Design review of the part shown in the three views and the two pictorial views. Dimensions are in mm from the part's minimum x, y and z. A direction names the side the tool comes from. Round coordinates to 2 decimals unless told otherwise and drop trailing zeros. Order: outer loops, then holes, each group sorted by start corner. A loop starts at its lowest first (then second) coordinate and runs counter-clockwise, first axis right, second up.
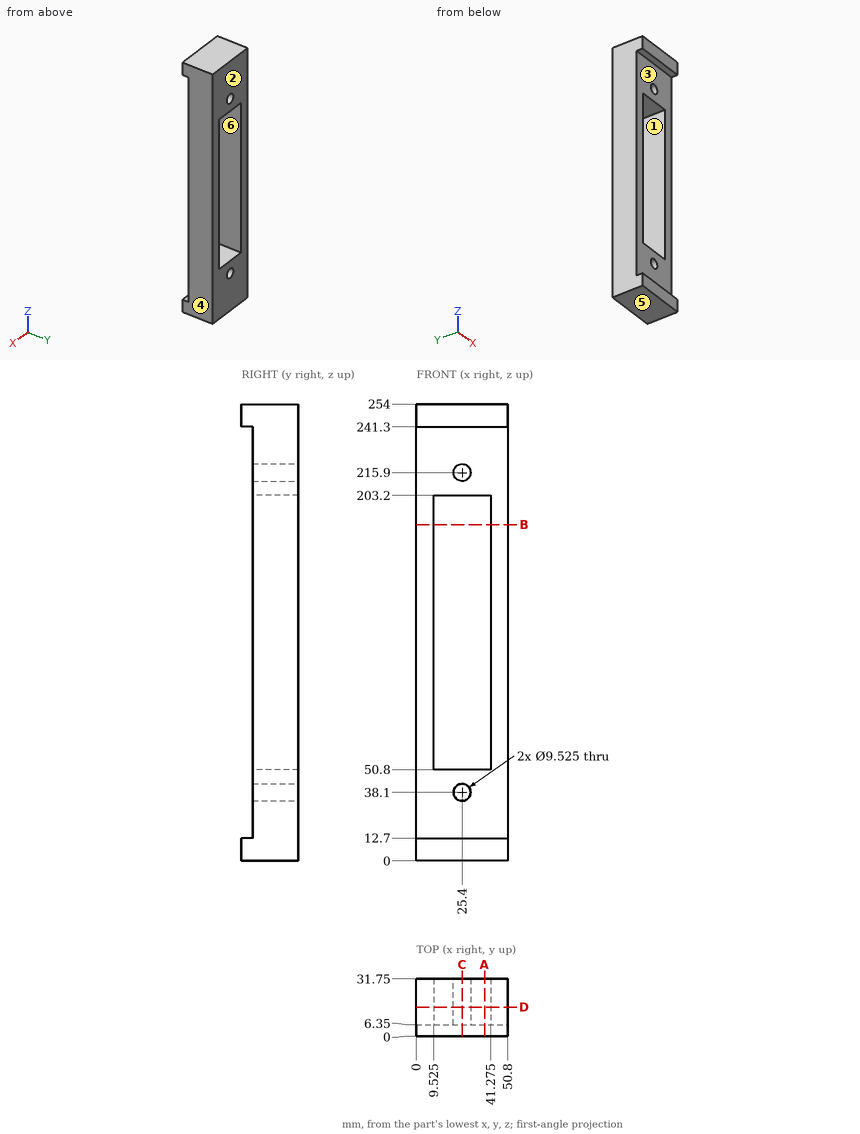
(1) Consider section B-B (z = 187). Write out the cut boundary in (x, y) (3 decimals).
Data:
outline: (0, 6.35) - (9.525, 6.35) - (9.525, 31.75) - (0, 31.75) - close; (41.275, 6.35) - (50.8, 6.35) - (50.8, 31.75) - (41.275, 31.75) - close
(2) To check wall thickness, follow probe 1 along Z at (x, y) = (25, 13); probe 2 along Z at (x, y) = (25.4, 17); probe 3 along Z at (x, y) = (16, 9.5). State the ranges of each line that lie inside material, in increasing order.
Data:
probe 1: z = 0 to 33.35, 42.85 to 50.8, 203.2 to 211.15, 220.65 to 254
probe 2: z = 0 to 33.34, 42.86 to 50.8, 203.2 to 211.14, 220.66 to 254
probe 3: z = 0 to 50.8, 203.2 to 254
(3) Draft analysis for pull direction Z (two halves, no side actions). For the marked faces 4, 5 and 6, state which applies: pulls with the +Z half, pulls with the -Z half, needs draft (parallel to the pull), parting line crosses it, or undercut.
Data:
face 4: needs draft
face 5: pulls with the -Z half
face 6: undercut
(4) Consider section D-D (y = 16). Write out the cut boundary in (x, z) (1 decimal), and give its area (3 significant figures).
Data:
outline: (0, 0) - (50.8, 0) - (50.8, 254) - (0, 254) - close; hole (9.5, 50.8) - (41.3, 50.8) - (41.3, 203.2) - (9.5, 203.2) - close; hole circle Ø9.5 at (25.4, 38.1); hole circle Ø9.5 at (25.4, 215.9)
area: 7,920 mm2
(5) Insertion check: pin 1 (12.5 mm diameter, centred on x = 25.4, z = 215.9, fed in from -Y); pin 2 (8.5 mm diameter, centred on x = 25.4, z = 38.1, fed in from -Y). Each pin has a flat end and moves straight along its axis. Give the tip position at first contact, or say it passes through.
Data:
pin 1: stops at y = 6.35
pin 2: passes through
(6) For the marked faces 1, 2 and 3, list the 3-axis set-ups (+Z, -Z, +X, -X, +Y, -Y) from which the entire face can be reached by the end or side of a thin tool; tool diameter is ignored.
Data:
face 1: +Y, -Y
face 2: +Z, -Z, +X, -X, +Y
face 3: +X, -X, -Y
(7) Consider section C-C (x = 25.4). Write out the cut boundary in (y, z), and give its area (3 significant figures).
Data:
outline: (0, 0) - (31.75, 0) - (31.75, 33.34) - (6.35, 33.34) - (6.35, 12.7) - (0, 12.7) - close; (0, 241.3) - (6.35, 241.3) - (6.35, 220.66) - (31.75, 220.66) - (31.75, 254) - (0, 254) - close; (6.35, 42.86) - (31.75, 42.86) - (31.75, 50.8) - (6.35, 50.8) - close; (6.35, 203.2) - (31.75, 203.2) - (31.75, 211.14) - (6.35, 211.14) - close
area: 2,260 mm2
(8) Consider section A-A (x = 38). Write out the cut boundary in (y, z), and give its area (3 significant figures).
Data:
outline: (0, 0) - (31.75, 0) - (31.75, 50.8) - (6.35, 50.8) - (6.35, 12.7) - (0, 12.7) - close; (0, 241.3) - (6.35, 241.3) - (6.35, 203.2) - (31.75, 203.2) - (31.75, 254) - (0, 254) - close
area: 2,740 mm2
